```python
from build123d import *

# Parameters (mm, degrees)
BOSS_EXTRUDE1_DEPTH = 1.5


with BuildPart() as part:
    # Sketch1 → Boss-Extrude1 (new, symmetric)
    with BuildSketch(Plane(origin=(0, 0, 0), x_dir=(1, 0, 0), z_dir=(0, 1, 0))):
        Polygon((49.5, 100), (40.5, 100), (40.5, 97), (31.5, 97), (31.5, 100), (22.5, 100), (22.5, 97), (13.5, 97), (13.5, 100), (4.5, 100), (4.5, 97), (-4.5, 97), (-4.5, 100), (-13.5, 100), (-13.5, 97), (-22.5, 97), (-22.5, 100), (-31.5, 100), (-31.5, 97), (-40.5, 97), (-40.5, 100), (-49.5, 100), (-49.5, 97), (-57, 97), (-57, 85.5), (-60, 85.5), (-60, 76.5), (-57, 76.5), (-57, 67.5), (-60, 67.5), (-60, 58.5), (-57, 58.5), (-57, 49.5), (-60, 49.5), (-60, 40.5), (-57, 40.5), (-57, 31.5), (-60, 31.5), (-60, 22.5), (-57, 22.5), (-57, 13.5), (-60, 13.5), (-60, 4.5), (-57, 4.5), (-57, -4.5), (-60, -4.5), (-60, -13.5), (-57, -13.5), (-57, -22.5), (-60, -22.5), (-60, -31.5), (-57, -31.5), (-57, -40.5), (-60, -40.5), (-60, -49.5), (-57, -49.5), (-57, -58.5), (-60, -58.5), (-60, -67.5), (-57, -67.5), (-57, -76.5), (-60, -76.5), (-60, -85.5), (-57, -85.5), (-57, -97), (-49.5, -97), (-49.5, -100), (-40.5, -100), (-40.5, -97), (-31.5, -97), (-31.5, -100), (-22.5, -100), (-22.5, -97), (-13.5, -97), (-13.5, -100), (-4.5, -100), (-4.5, -97), (4.5, -97), (4.5, -100), (13.5, -100), (13.5, -97), (22.5, -97), (22.5, -100), (31.5, -100), (31.5, -97), (40.5, -97), (40.5, -100), (49.5, -100), (49.5, -97), (57, -97), (57, -85.5), (60, -85.5), (60, -76.5), (57, -76.5), (57, -67.5), (60, -67.5), (60, -58.5), (57, -58.5), (57, -49.5), (60, -49.5), (60, -40.5), (57, -40.5), (57, -31.5), (60, -31.5), (60, -22.5), (57, -22.5), (57, -13.5), (60, -13.5), (60, -4.5), (57, -4.5), (57, 4.5), (60, 4.5), (60, 13.5), (57, 13.5), (57, 22.5), (60, 22.5), (60, 31.5), (57, 31.5), (57, 40.5), (60, 40.5), (60, 49.5), (57, 49.5), (57, 58.5), (60, 58.5), (60, 67.5), (57, 67.5), (57, 76.5), (60, 76.5), (60, 85.5), (57, 85.5), (57, 97), (49.5, 97), align=None)
    extrude(amount=BOSS_EXTRUDE1_DEPTH, both=True)


solid = part.part
```
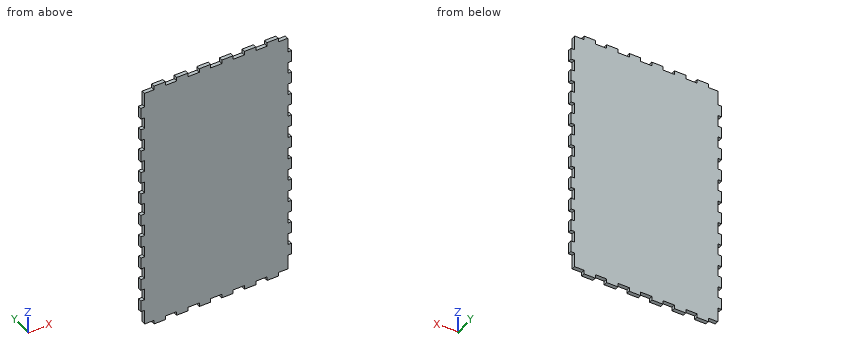
Here's how the part is built. I have some questions about the finished solid (model axes, mm). Round coordinates to 2 decimals unless told otherwise and drop trailing zeros. Write each loop counter-clockwise with the first axis right and the second up, starting at its lowest first coordinate (ties: lowest second). Pieces come first, ordered by that corner, then holes.
Q1. If we section it at B-B on z = -18.5: Write out the boundary of the cut face in (x, y), plus the area to 3 significant figures.
Q2. If we section it at A-A on x = -17: Write out the boundary of the cut face in (y, z), plus the area to 3 significant figures.
Q3. Will these pins go through, and if not, where does the flat tip stop? P1, Ø0.9, axis at x = 58, y = 0.5, coming from the -Z side; P2, Ø0.9, axis at y = 0.5, z = -98, coming from the -X side; P3, Ø1.5, axis at y = -0.5, z = 91.5, coming from the -X side.
Q4. Please list where these lines run through material, in increasing order: probe 1 along X at (y, z) = (-1.1, 19); probe 2 along Z at (x, y) = (-36, -0.5).
Answer below:
1. outline: (-57, -1.5) - (57, -1.5) - (57, 1.5) - (-57, 1.5) - close
1. area: 342 mm2
2. outline: (-1.5, -97) - (1.5, -97) - (1.5, 97) - (-1.5, 97) - close
2. area: 582 mm2
3. P1: stops at z = -85.5
3. P2: stops at x = -49.5
3. P3: stops at x = -57
4. probe 1: x = -57 to 57
4. probe 2: z = -97 to 97
